Can you work these out from the model? Positions are in its coordinate system, mm. Face numbers are marked on the shaded views. A direction names the side the tool comes from. Give positions to 0.01 mm unless a question says otherwise; leave off trailing zeros. Order: outer loops, then holes, each group sorted by start corner. A loop starts at its lowest first (then second) coordinate and runs counter-clockwise, first axis right, second up.
Item 1: If I drill on line 1 along Y through (x, z) = (29, 18); line 2 along X through (y, z) = (-11.5, 24); line 3 along X through (y, z) = (-1, 15.5), over which ranges is the centre line in solid material (lowest first)?
Item 2: I want a section at B-B, the plane x = 55. Write out the boundary of the cut face in (y, z).
Item 3: I'm going to push flat-ended pins straight in: pin 1 Ø12 at (x, z) = (-5, 21.5) entering from +Y; pin 2 Ø7.5 at (x, y) = (-44.5, -3.5) entering from +Z; pin 3 Ø5.5 at (x, z) = (53.5, 9.5) entering from +Y; pin 4 Ø12.5 at (y, z) = (11, 37.5) entering from +X. Where does each tip first touch, or does it pass through?
Item 4: I want a section at A-A, the plane z = 36.5. Write out the boundary of the cut face in (x, y), then the cut area to 3 significant figures.
Item 5: I want a section at D-D, the plane z = 6. Write out the boundary of the cut face in (x, y).
Item 6: I want a section at C-C, the plane y = -13. Write out the boundary of the cut face in (x, z), then the cut area to 3 significant figures.
Item 7: Which directions (+Z, -Z, +X, -X, +Y, -Y) give clear straight access to the entire face, cutting with the end or side of a thin tool? Please do the marked faces 1, 2 and 3.
Item 8: If we mould it in two halves opening along Y, with no side actions, what happens to the marked faces 4, 5 and 6? For each: +Y half, -Y half, draft (parallel to the pull), parting line (faces both ways), or undercut.
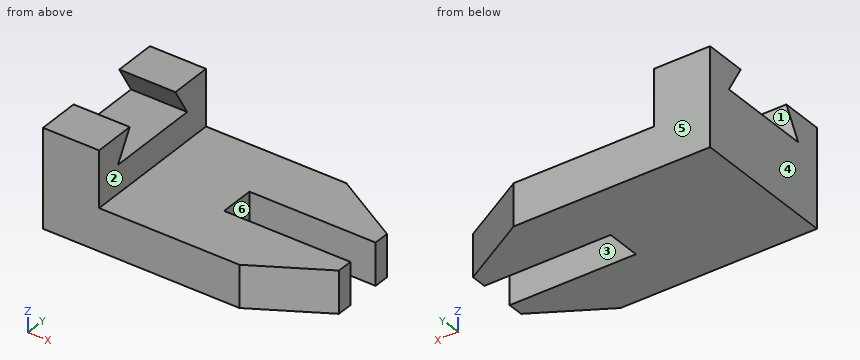
```python
from build123d import *

# Parameters (mm, degrees)
F0_W     = 120.65
F0_H     = 66.548
F1_DEPTH = 44.45
F2_W     = 95.25
F2_H     = 25.4
F3_DEPTH = 182.372
F5_DEPTH = 80.518
F7_DEPTH = 103.632
F9_DEPTH = 44.196


with BuildPart() as f1:
    # F0 (on Top) → F1 (new body)
    with BuildSketch(Plane.XY):
        with Locations((8.846484, 5.5548)):
            Rectangle(F0_W, F0_H)
    extrude(amount=F1_DEPTH)

    # F2 (on face) → F3 (cut)
    with BuildSketch(Plane.XZ.offset(27.7192)):
        with Locations((21.546484, 31.75)):
            Rectangle(F2_W, F2_H)
    extrude(amount=-F3_DEPTH, mode=Mode.SUBTRACT)

    # F4 (on face) → F5 (cut)
    with BuildSketch(Plane.XY.offset(19.05)):
        Polygon((69.171484, 5.5548), (69.171484, 13.4288), (12.021484, 13.4288), (12.021484, 5.5548), (12.021484, -2.3192), (69.171484, -2.3192), align=None)
    extrude(amount=-F5_DEPTH, mode=Mode.SUBTRACT)

    # F6 (on face) → F7 (cut)
    with BuildSketch(Plane.YZ.offset(-26.078516)):
        Polygon((5.5548, 44.45), (-8.6692, 44.45), (-16.001548, 31.75), (-8.6692, 31.75), (5.5548, 31.75), (19.7788, 31.75), (27.111149, 31.75), (19.7788, 44.45), align=None)
    extrude(amount=-F7_DEPTH, mode=Mode.SUBTRACT)

    # F8 (on face) → F9 (cut)
    with BuildSketch(Plane.XY.offset(19.05)):
        Polygon((37.421484, -27.7192), (69.171484, -27.7192), (69.171484, -9.388329), align=None)
        Polygon((69.171484, 20.497929), (69.171484, 38.8288), (37.421484, 38.8288), align=None)
    extrude(amount=-F9_DEPTH, mode=Mode.SUBTRACT)


solid = f1.part
```
Results list:
1. line 1: y = -27.72 to -2.32, 13.43 to 38.83
1. line 2: x = -51.48 to -26.08
1. line 3: x = -51.48 to 12.02
2. outline: (-17.57, 0) - (-2.32, 0) - (-2.32, 19.05) - (-17.57, 19.05) - close; (13.43, 0) - (28.68, 0) - (28.68, 19.05) - (13.43, 19.05) - close
3. pin 1: stops at y = 38.83
3. pin 2: stops at z = 31.75
3. pin 3: stops at y = 31.13
3. pin 4: stops at x = -26.08
4. outline: (-51.48, -27.72) - (-26.08, -27.72) - (-26.08, -13.26) - (-51.48, -13.26) - close; (-51.48, 24.37) - (-26.08, 24.37) - (-26.08, 38.83) - (-51.48, 38.83) - close
4. area: 735 mm2
5. outline: (-51.48, -27.72) - (37.42, -27.72) - (69.17, -9.39) - (69.17, -2.32) - (12.02, -2.32) - (12.02, 13.43) - (69.17, 13.43) - (69.17, 20.5) - (37.42, 38.83) - (-51.48, 38.83) - close
6. outline: (-51.48, 0) - (62.92, 0) - (62.92, 19.05) - (-26.08, 19.05) - (-26.08, 31.75) - (-51.48, 31.75) - close; (-51.48, 36.95) - (-26.08, 36.95) - (-26.08, 44.45) - (-51.48, 44.45) - close
6. area: 2,690 mm2
7. face 1: +X, -X
7. face 2: +Z, +X, +Y, -Y
7. face 3: +Z, -Z, +X
8. face 4: draft
8. face 5: +Y half
8. face 6: undercut
